```python
from build123d import *

# Parameters (mm, degrees)
F1_DEPTH = 25
F3_D     = 5
F4_R     = 5


with BuildPart() as f1:
    # F0 (on Top) → F1 (new body)
    with BuildSketch(Plane.XY):
        with BuildLine():
            Line((10, -5), (10, 0))
            ThreePointArc((10, 0), (0, 10), (-10, 0))
            Line((-10, 0), (-10, -25))
            Line((-10, -25), (5, -25))
            Line((5, -25), (5, -5))
            Line((5, -5), (10, -5))
        make_face()
    extrude(amount=F1_DEPTH)

    # F3 (through all)
    with Locations(Plane(origin=(-10, 0, 0), x_dir=(0, -1, 0), z_dir=(-1, 0, 0))):
        with Locations((13.501376, 13.991057)):
            Hole(F3_D / 2)

    # F4
    f4_edges = [f1.edges().sort_by_distance(p)[0] for p in [
        (-10, -25, 12.5),
    ]]
    fillet(f4_edges, radius=F4_R)


solid = f1.part
```
Here's how the part is built. I have some questions about the finished solid (model axes, mm). A direction names the side the tool comes from. Coordinates: 2 decimals unless noted, no trailing zeros. Write each loop counter-clockwise with the first axis right and the second up, starting at its lowest first coordinate (ties: lowest second). Pieces come first, ordered by that corner, then holes. Notation, with made-up numbers: M -27.5,79.5 L -18.5,79.5 A18 ccw -18.5,103.5 Z; hole C 7.5,-37 d3. An arc over 180 degrees is marked long. Answer as CSV lines item,"result". Start each with the question number.
Q1. If we mould it in two halves opening along Z, with no side actions, what happens to faces 3 (the flat face through (0, -7, 25)), 4 (the cylindrical face through (-2.395, -11.192, 13.034)), 5 (the flat face through (0, -25, 12))? For each: pulls with the +Z half, pulls with the -Z half, needs draft (parallel to the pull), parting line crosses it, or undercut.
Q2. Suppose I cut it at C-C, the plane y = -16.5. List the corners of the cut face in (x, z) for me.
Q3. Suppose I cut it at A-A, the plane z = 18.25. List the corners of the cut face in (x, y) for me, then the cut area to 3 significant figures.
Q4. Suppose I cut it at B-B, the plane x = 2.25. List the corners of the cut face in (y, z) for me.
Q5. I need wall thicknesses on probe 1 along X at (y, z) = (-14, 20.5); probe 2 along Y at (x, z) = (0.5, 16); probe 3 along Y at (x, z) = (-7, 14.75). Which ranges of each line are inside material? Lowest first, please. Write a range as [from, to].
Q6. For faces 1 (the flat face through (-10, -10, 12)), 2 (the flat face through (7, -5, 12)), which set-ups out of +Z, -Z, +X, -X, +Y, -Y let a thin tool reach every point of the face, with its end or its side?
Q7. Will these pins go through, and if not, where does the flat tip stop? pin 1 Ø10 at (y, z) = (-15, 16) entering from +X; pin 2 Ø6 at (x, z) = (8, 17) entering from +Y; pin 3 Ø1.5 at (x, z) = (8, 13) entering from -Y.
Q8. Suppose I cut it at D-D, the plane x = 0. List the corners of the cut face in (y, z) for me, then the cut area to 3 significant figures.
Entries:
1,face 3,"pulls with the +Z half"
1,face 4,"undercut"
1,face 5,"needs draft"
2,outline,"M -10,0 L 5,0 L 5,25 L -10,25 Z"
3,outline,"M -10,-20 A5 ccw -5,-25 L 5,-25 L 5,-5 L 10,-5 L 10,0 A10 ccw -10,0 Z"
3,area,"552 mm²"
4,outline,"M -25,0 L 9.74,0 L 9.74,25 L -25,25 Z; hole C -13.5,13.99 d5"
5,probe 1,"x = [-10, 5]"
5,probe 2,"y = [-25, -14.99], [-12.01, 9.99]"
5,probe 3,"y = [-24.58, -15.88], [-11.12, 7.14]"
6,face 1,"+Z, -Z, -X, +Y, -Y"
6,face 2,"+Z, -Z, +X, -Y"
7,pin 1,"stops at x = 5"
7,pin 2,"stops at y = 8.66"
7,pin 3,"stops at y = -5"
8,outline,"M -25,0 L 10,0 L 10,25 L -25,25 Z; hole C -13.5,13.99 d5"
8,area,"855 mm²"
